```python
from build123d import *

# Parameters (mm, degrees)
F0_R     = 2
F0_W     = 37
F0_H     = 37
F1_DEPTH = 3


with BuildPart() as f1:
    # F0 (on Front) → F1 (new body)
    with BuildSketch(Plane.XZ):
        with BuildLine():
            Line((65, 42), (-65, 42))
            ThreePointArc((-65, 42), (-68.535534, 40.535534), (-70, 37))
            Line((-70, 37), (-70, -37))
            ThreePointArc((-70, -37), (-68.535534, -40.535534), (-65, -42))
            Line((-65, -42), (65, -42))
            ThreePointArc((65, -42), (68.535534, -40.535534), (70, -37))
            Line((70, -37), (70, 37))
            ThreePointArc((70, 37), (68.535534, 40.535534), (65, 42))
        make_face()
        with Locations((-63, -32)):
            Circle(F0_R, mode=Mode.SUBTRACT)
        with Locations((63, -32)):
            Circle(F0_R, mode=Mode.SUBTRACT)
        with Locations((26.5, -6.5)):
            Rectangle(F0_W, F0_H, mode=Mode.SUBTRACT)
        with Locations((-26.5, 6.5)):
            Rectangle(F0_W, F0_H, mode=Mode.SUBTRACT)
        with Locations((-63, 32)):
            Circle(F0_R, mode=Mode.SUBTRACT)
        with Locations((0, 27)):
            Circle(F0_R, mode=Mode.SUBTRACT)
        with Locations((63, 32)):
            Circle(F0_R, mode=Mode.SUBTRACT)
    extrude(amount=F1_DEPTH)


solid = f1.part
```
CAD build for the part. Positions are in the model's coordinates, mm. A direction names the side the tool comes from. Give positions to 0.01 mm unless a question says otherwise; leave off trailing zeros. Order: outer loops, then holes, each group sorted by start corner. A loop starts at its lowest first (then second) coordinate and runs counter-clockwise, first axis right, second up. Notation, with made-up numbers: M -29,-9.75 L 14,-9.75 A32 ccw 14,17.25 Z; hole C -33.75,44.5 d7. An arc over 180 degrees is marked long. Put each result on its own line as item: value. Start each with the question number.
(1) Saw through at A-A, the plane z = 32. Write the cut outline in (x, y), then the cut area to 3 significant figures.
(2) Mould opens along X. For faces 1 (the flat face through (-1, 0, 1)), 2 (the cylindrical face through (63, -1, 30)), 3 (the cylindrical face through (-68, -1, 41)), 4 (the flat face through (70, -1, -1)) say: +X half, -X half, draft (parallel to the pull), parting line (faces both ways), or undercut.
(3) Which spindle directions (+Z, -Z, +X, -X, +Y, -Y) get a long thin tool onto all of the face, cutting with end or side? Do faces 5 (the flat face through (-1, -3, 1)), 6 (the flat face through (45, -1, -7)). Say none if no direction does.
(4) Saw through at C-C, the plane z = -23. Write the cut outline in (x, y).
(5) Saw through at B-B, the plane x = 37.5. Write the cut outline in (y, z).
(6) Drill centre lines: line 1 along Z through (x, y) = (63, -0.75); line 2 along X through (y, z) = (-1.7, -3.5); line 3 along Z through (x, y) = (-41, -1.35). Where is each one in solid material? Low to high.
(7) Saw through at D-D, the plane x = 63. Write the cut outline in (y, z).
Check result:
1. outline: M -70,-3 L -65,-3 L -65,0 L -70,0 Z; M -61,-3 L 61,-3 L 61,0 L -61,0 Z; M 65,-3 L 70,-3 L 70,0 L 65,0 Z
1. area: 396 mm2
2. face 1: draft
2. face 2: undercut
2. face 3: -X half
2. face 4: +X half
3. face 5: +Z, -Z, +X, -X, -Y
3. face 6: +Y, -Y
4. outline: M -70,-3 L 8,-3 L 8,0 L -70,0 Z; M 45,-3 L 70,-3 L 70,0 L 45,0 Z
5. outline: M -3,-42 L 0,-42 L 0,-25 L -3,-25 Z; M -3,12 L 0,12 L 0,42 L -3,42 Z
6. line 1: z = -42 to -34, -30 to 30, 34 to 42
6. line 2: x = -70 to -45, -8 to 8, 45 to 70
6. line 3: z = -42 to -12, 25 to 42
7. outline: M -3,-42 L 0,-42 L 0,-34 L -3,-34 Z; M -3,-30 L 0,-30 L 0,30 L -3,30 Z; M -3,34 L 0,34 L 0,42 L -3,42 Z
